Verification items for the finished model (mm, model axes). A direction names the side the tool comes from. Coordinates: 2 decimals unless noted, no trailing zeros. Write each loop counter-clockwise with the first axis right and the second up, starting at its lowest first coordinate (ties: lowest second). Pieces come first, ordered by that corner, then holes. Notation, with made-up numbers: M -13.75,31.25 L 24.25,31.25 A29 cw 24.25,54.25 Z; hole C -24,62 d6. An arc over 180 degrees is marked long. Answer in a Markdown table with one row per item.
from build123d import *

# Parameters (mm, degrees)
SKETCH_9_W          = 1
SKETCH_9_H          = 4
SKETCH_10_R         = 5.1
CUT_EXTRUDE_1_DEPTH = 10


with BuildPart() as part:
    # 草图7 → 旋转1 (revolve)
    with BuildSketch(Plane.XY, mode=Mode.PRIVATE) as revolve_1_sk:
        with BuildLine():
            Line((-5, 4), (-5, -4))
            Line((-5, -4), (-5, -7))
            Line((-5, -7), (-12, -7))
            Line((-12, -7), (-12, -5))
            ThreePointArc((-12, -5), (-7, 0), (-12, 5))
            Line((-12, 5), (-12, 7))
            Line((-12, 7), (-5, 7))
            Line((-5, 7), (-5, 4))
        make_face()
    revolve(revolve_1_sk.sketch.rotate(Axis((0, 0, 0), (0, 1, 0)), 270), axis=Axis((0, 0, 0), (0, 1, 0)))

    # 草图9 → 旋转2 (revolve)
    with BuildSketch(Plane.XY, mode=Mode.PRIVATE) as revolve_2_sk:
        with Locations((-4.5, 5)):
            Rectangle(SKETCH_9_W, SKETCH_9_H)
        with Locations((-4.5, -5)):
            Rectangle(SKETCH_9_W, SKETCH_9_H)
    revolve(revolve_2_sk.sketch.rotate(Axis((0, 0, 0), (0, 1, 0)), 270), axis=Axis((0, 0, 0), (0, 1, 0)))

    # 草图10 → 切除-拉伸1 (cut)
    with BuildSketch(Plane.XZ.offset(7)):
        with Locations(Location((0, 0, 0), (0, 0, 270))):
            Circle(SKETCH_10_R)
    extrude(amount=-CUT_EXTRUDE_1_DEPTH, mode=Mode.SUBTRACT)


solid = part.part
1) Release check for a two-part mould opening along X. For faces 1 (the face through (3, 3, 3)), 2 (the face through (2, -7, -5)), 3 (the face through (-3.604, 6.014, -11.446)) record: +X half, -X half, draft (parallel to the pull), parting line (faces both ways), or undercut.
Response values:
| item | result |
|---|---|
| face 1 | undercut |
| face 2 | draft |
| face 3 | parting line |
2) Sectioned sample at A-A (z = 0). Record the cut outline in (x, y).
Response values:
| item | result |
|---|---|
| outline | M -12,-7 L -5.1,-7 L -5.1,3 L -4,3 L -4,7 L -12,7 L -12,5 A5 cw -12,-5 Z; M 4,3 L 5.1,3 L 5.1,-7 L 12,-7 L 12,-5 A5 cw 12,5 L 12,7 L 4,7 Z |
3) Sectioned sample at C-C (y = -6). Record the cut outline in (x, z), then the cut area to 3 significant figures.
Response values:
| item | result |
|---|---|
| outline | C 0,0 d24; hole C 0,0 d10.2 |
| area | 371 mm² |
4) Tool access check on faces 4 (the face through (1.532, -2.07, -4.864)), 5 (the face through (-3, 7, 3)). Record the directions out of +Z, -Z, +X, -X, +Y, -Y that give a thin tool (end or side, any length) a straight path to the whole face; none if there is none.
Response values:
| item | result |
|---|---|
| face 4 | -Y |
| face 5 | +Z, -Z, +X, -X, +Y |
5) Sectioned sample at B-B (x = 0). Record the cut outline in (y, z), then the cut area to 3 significant figures.
Response values:
| item | result |
|---|---|
| outline | M -7,-12 L -5,-12 A5 cw 5,-12 L 7,-12 L 7,-4 L 3,-4 L 3,-5.1 L -7,-5.1 Z; M -7,5.1 L 3,5.1 L 3,4 L 7,4 L 7,12 L 5,12 A5 cw -5,12 L -7,12 Z |
| area | 123 mm² |
6) Sectioned sample at D-D (y = -2.25). Record the cut outline in (x, z), then the cut area to 3 significant figures.
Response values:
| item | result |
|---|---|
| outline | C 0,0 d15.07; hole C 0,0 d10.2 |
| area | 96.6 mm² |
7) Thickness scan on L1, parallel to X at y = -2, z = 0; L2, parallel to Y at x = 6, z = -4.5; L3, parallel to X at y = -1.5, z = 3. Record the ranges inside material, lowest first. Write a range as [from, to].
Response values:
| item | result |
|---|---|
| L1 | x = [-7.42, -5.1], [5.1, 7.42] |
| L2 | y = [-7, -2.18], [2.18, 7] |
| L3 | x = [-6.58, -4.12], [4.12, 6.58] |
8) Depth check by flat-ended pin: pin 1 (3 mm diameter, centred on x = 0, z = -4, fed in from -Y); pin 2 (8 mm diameter, centred on x = -5, y = -3.5, fed in from +Z); pin 3 (2 mm diameter, centred on y = 5.5, z = 4.5, fed in from +X). Enter the tip coordinate at first touch or a pass-through.
Response values:
| item | result |
|---|---|
| pin 1 | stops at y = -7 |
| pin 2 | stops at z = 11.93 |
| pin 3 | stops at x = 11.48 |
